Design review of the part built by this model. Coordinates are the model's own, in mm. A direction names the side the tool comes from. Round coordinates to 2 decimals unless told otherwise and drop trailing zeros. Loops run counter-clockwise (first coordinate to the right, second up) from the corner with the lowest first, then second, coordinate; pieces in that order, holes last. Notation, with made-up numbers: (-8.5, 74) - (20.5, 74) arc R23 ccw to (20.5, 101) - close; hole circle Ø5 at (20, 6). An arc over 180 degrees is marked (long way). Return JSON: item names as keys, results as strings. Group by question number.
(1) We need section C-C, the plane z = -27.5. Write out the cut boundary in (x, y), and give its area (3 significant figures).
(2) Clearance check with flat-ended pins moving along their axes: pin 1 (5.5 mm diameter, centred on x = 17.5, z = 27, fed in from +Y); pin 2 (6 mm diameter, centred on x = 5.08, z = 21.22, fed in from +Y). State where each tip first meets the part, or that it passes through.
(3) For faces 4 (the flat face through (0, -4, -1)), 5 (the cylindrical face through (18.83, -1.126, 20.037)), list the 3-axis set-ups (+Z, -Z, +X, -X, +Y, -Y) from which the entire face can be reached by the end or side of a thin tool; tool diameter is ignored.
(4) We need section A-A, the plane y = -6.5. Write out the cut boundary in (x, z), and give its area (3 significant figures).
(5) We need section B-B, the plane x = 19.05. Write out the cut boundary in (y, z).
(6) Wall thickness on L1, parallel to Z at x = 19, y = -8; L2, parallel to Z at x = 18, y = -6; L3, parallel to X at y = -4.75, z = 25.5: over which ranges is each line inside the solid? List them lowest first. Write a range as [from, to].
(7) The part is to be moulded in two halves that separate along Z. For faces 1 (the flat face through (19, -4, 31.383)), 2 (the flat face through (19, -8.705, -1)), 3 (the cylindrical face through (4.98, -3.64, 23.47)), say which applies: pulls with the +Z half, pulls with the -Z half, needs draft (parallel to the pull), parting line crosses it, or undercut.
(8) We need section D-D, the plane y = -1.25. Write out the cut boundary in (x, z).
Autodesk Inventor part; units mm, degrees
ref_plane "YZ Plane" through (0, 0, 0) normal (1, 0, 0) x (0, 1, 0)
ref_plane "XZ Plane" through (0, 0, 0) normal (0, 1, 0) x (-1, 0, 0)
ref_plane "XY Plane" through (0, 0, 0) normal (0, 0, 1) x (1, 0, 0)
sketch "Sketch1" plane through (0, 0, 0) normal (1, 0, 0) x (0, 1, 0)
  line L0 (1.2948, 31.3833) -> (-8.7052, 31.3833)
  line L1 (-8.7052, 31.3833) -> (-8.7052, -33.6153)
  line L2 (-8.7052, -33.6153) -> (1.2948, -33.6153)
  line L3 (1.2948, -33.6153) -> (1.2948, 31.3833)
  point P0 (0, 0)
  dimension "d0" = 64.9986
  dimension "d1" = 10
extrude "Extrusion1" add sketch "Sketch1" along normal blind 38.1
sketch "Sketch2" plane through (0, 1.2948, 31.3833) normal (0, 1, 0) x (1, 0, 0)
  line L0 (38.1, 64.9986) -> (38.1, 0)
  line L1 (0, 0) -> (38.1, 0)
  line L2 (0, 64.9986) -> (38.1, 64.9986)
  point P0 (0, 31.3833)
  point P1 (19.05, 5)
  point P2 (19.05, 59.9986)
  dimension "d4" = 0
  dimension "d5" = 19.05
  dimension "d6" = 5
  dimension "d7" = 5
hole "Hole1" at (19.05, 1.2948, 26.3833) at (19.05, 1.2948, -28.6153) direction (0, -1, 0) diameter 6.7564 end through all counterbore diameter 12.7 counterbore depth 4.7752
sketch "Sketch3" plane through (0, -8.7052, -33.6153) normal (0, -1, 0) x (1, 0, 0)
  line L0 (38.1, 64.9986) -> (38.1, 0)
  line L1 (0, 64.9986) -> (0, 0)
  line L2 (0, 64.9986) -> (38.1, 64.9986)
  line L3 (0, 0) -> (38.1, 0)
  point P0 (0, 33.6153)
  point P1 (5.08, 54.8386)
  point P2 (5.08, 10.16)
  dimension "d16" = 5.08
  dimension "d24" = 10.16
  dimension "d25" = 10.16
  dimension "d26" = 5.08
hole "Hole2" at (5.08, -8.7052, 21.2233) at (5.08, -8.7052, -23.4553) direction (0, 1, 0) diameter 4.4958 end through all
properties part number "LidarV4MountLongPlate"
Solutions:
{
 "1": {"outline": "(0, -8.71) - (15.86, -8.71) - (15.86, -3.48) - (12.8, -3.48) - (12.8, 1.29) - (0, 1.29) - close; (22.24, -8.71) - (38.1, -8.71) - (38.1, 1.29) - (25.3, 1.29) - (25.3, -3.48) - (22.24, -3.48) - close", "area": "288 mm^2"},
 "2": {"pin 1": "y = -3.48", "pin 2": "y = 1.29"},
 "3": {"face 4": "+Z, -Z, -X, +Y, -Y", "face 5": "+Y"},
 "4": {"outline": "(0, -33.62) - (38.1, -33.62) - (38.1, 31.38) - (0, 31.38) - close; hole circle Ø4.5 at (5.08, -23.46); hole circle Ø4.5 at (5.08, 21.22); hole circle Ø6.76 at (19.05, -28.62); hole circle Ø6.76 at (19.05, 26.38)", "area": "2,370 mm^2"},
 "5": {"outline": "(-8.71, -33.62) - (-3.48, -33.62) - (-3.48, -31.99) - (-8.71, -31.99) - close; (-8.71, -25.24) - (-3.48, -25.24) - (-3.48, -22.27) - (1.29, -22.27) - (1.29, 20.03) - (-3.48, 20.03) - (-3.48, 23.01) - (-8.71, 23.01) - close; (-8.71, 29.76) - (-3.48, 29.76) - (-3.48, 31.38) - (-8.71, 31.38) - close"},
 "6": {"L1": "[-33.62, -31.99], [-25.24, 23.01], [29.76, 31.38]", "L2": "[-33.62, -31.83], [-25.4, 23.17], [29.59, 31.38]", "L3": "[0, 15.79], [22.31, 38.1]"},
 "7": {"face 1": "pulls with the +Z half", "face 2": "needs draft", "face 3": "undercut"},
 "8": {"outline": "(0, -33.62) - (15.14, -33.62) arc R6.35 cw (long way) to (22.96, -33.62) - (38.1, -33.62) - (38.1, 31.38) - (22.96, 31.38) arc R6.35 cw (long way) to (15.14, 31.38) - (0, 31.38) - close; hole circle Ø4.5 at (5.08, -23.46); hole circle Ø4.5 at (5.08, 21.22)"}
}
